Design review of the part built by this model. Coordinates are the model's own, in mm. Face numbers are marked on the shaded views. Give positions to 0.01 mm unless a question says otherwise; leave off trailing zeros. Write each loop counter-clockwise with the first axis right and the second up, starting at its lowest first coordinate (ties: lowest second). Pieces come first, ordered by that corner, then holes. Notation, with made-up numbers: M 40.25,43 L 49.25,43 A23 cw 49.25,60 Z; hole C -35.5,-14.5 d6. An arc over 180 degrees is marked long. Use one line per item in the form item = value. Start each with the question number.
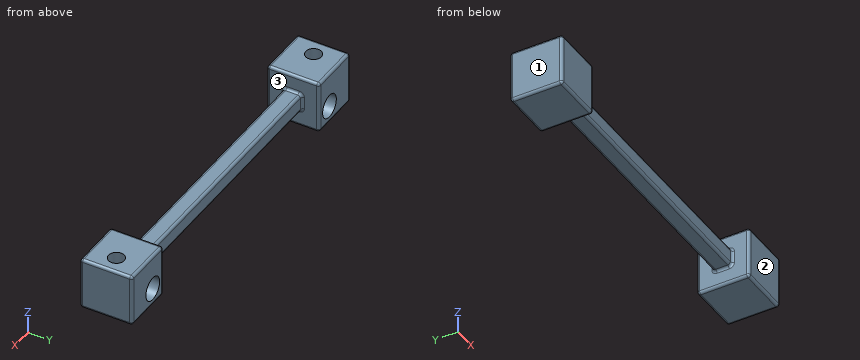
from build123d import *

# Parameters (mm, degrees)
BOSS_EXTRUDE1_START = -10
SKETCH1_W           = 30
SKETCH1_H           = 30
BOSS_EXTRUDE1_DEPTH = 30
SKETCH2_W           = 10
SKETCH2_H           = 10
BOSS_EXTRUDE2_DEPTH = 152.4
SKETCH3_W           = 6
SKETCH3_H           = 6
CUT_EXTRUDE1_DEPTH  = 152.4
SKETCH4_R           = 6.7
CUT_EXTRUDE2_DEPTH  = 15
SKETCH5_R           = 4.5
CUT_EXTRUDE3_DEPTH  = 15
FILLET3_R           = 1.5


with BuildPart() as part:
    # Sketch1 → Boss-Extrude1 (new body)
    with BuildSketch(Plane(origin=(0, 0, 0), x_dir=(0, 0, -1), z_dir=(1, 0, 0)).offset(BOSS_EXTRUDE1_START)):
        with Locations((15, 15)):
            Rectangle(SKETCH1_W, SKETCH1_H)
    boss_extrude1 = extrude(amount=BOSS_EXTRUDE1_DEPTH)

    # Sketch2 → Boss-Extrude2 (add)
    with BuildSketch(Plane(origin=(20, 0, 0), x_dir=(0, 0, -1), z_dir=(1, 0, 0))):
        with Locations((15, 15)):
            Rectangle(SKETCH2_W, SKETCH2_H)
    extrude(amount=BOSS_EXTRUDE2_DEPTH)

    # Sketch3 → Cut-Extrude1 (cut)
    with BuildSketch(Plane(origin=(172.4, 0, 0), x_dir=(0, 0, -1), z_dir=(1, 0, 0))):
        with Locations((15, 15)):
            Rectangle(SKETCH3_W, SKETCH3_H)
    extrude(amount=-CUT_EXTRUDE1_DEPTH, mode=Mode.SUBTRACT)

    # Sketch4 → Cut-Extrude2 (cut)
    with BuildSketch(Plane(origin=(0, 30, 0), x_dir=(1, 0, 0), z_dir=(0, 1, 0))):
        with Locations(Location((10, 20, 0), (0, 0, 270))):
            Circle(SKETCH4_R)
    cut_extrude2 = extrude(amount=-CUT_EXTRUDE2_DEPTH, mode=Mode.SUBTRACT)

    # Sketch5 → Cut-Extrude3 (cut)
    with BuildSketch(Plane.XY):
        with Locations((0, 15)):
            Circle(SKETCH5_R)
    cut_extrude3 = extrude(amount=-CUT_EXTRUDE3_DEPTH, mode=Mode.SUBTRACT)

    # Mirror1: Boss-Extrude1, Cut-Extrude2, Cut-Extrude3 across plane
    add(boss_extrude1.mirror(Plane(origin=(96.2, 0, 0), x_dir=(0, 0, 1), z_dir=(1, 0, 0))))
    add(cut_extrude2.mirror(Plane(origin=(96.2, 0, 0), x_dir=(0, 0, 1), z_dir=(1, 0, 0))), mode=Mode.SUBTRACT)
    add(cut_extrude3.mirror(Plane(origin=(96.2, 0, 0), x_dir=(0, 0, 1), z_dir=(1, 0, 0))), mode=Mode.SUBTRACT)

    # Fillet3
    fillet3_edges = [part.edges().sort_by_distance(p)[0] for p in [
        (20, 30, -15),
        (20, 15, 0),
        (20, 0, -15),
        (-10, 30, -15),
        (20, 15, -30),
        (-10, 15, 0),
        (20, 15, -10),
        (96.2, 20, -10),
        (20, 10, -15),
        (96.2, 10, -10),
        (20, 15, -20),
        (96.2, 10, -20),
        (20, 20, -15),
        (96.2, 20, -20),
        (172.4, 15, -10),
        (172.4, 10, -15),
        (172.4, 15, -20),
        (172.4, 20, -15),
        (-10, 0, -15),
        (187.4, 0, 0),
        (172.4, 0, -15),
        (187.4, 0, -30),
        (172.4, 15, -30),
        (187.4, 30, -30),
        (202.4, 30, -15),
        (187.4, 30, 0),
        (202.4, 15, 0),
        (202.4, 0, -15),
        (202.4, 15, -30),
        (172.4, 15, 0),
        (172.4, 30, -15),
        (5, 0, 0),
        (5, 30, 0),
        (5, 30, -30),
        (5, 0, -30),
        (-10, 15, -30),
    ]]
    fillet(fillet3_edges, radius=FILLET3_R)


solid = part.part
1. Clearance check with flat-ended pins moving along their axes: pin 1 Ø2 at (x, z) = (20, -7) entering from +Y; pin 2 Ø1.8 at (x, z) = (123.5, -16) entering from -Y; pin 3 Ø4.5 at (x, y) = (1.5, 15) entering from +Z. State where each tip first meets the part, or that it passes through.
2. We need section A-A (y = 24.5). State the section outline as (x, z) points.
3. To check wall thickness, follow L1, parallel to X at y = 24.25, z = -20; L2, parallel to Y at x = 92, z = -14.5; L3, parallel to X at y = 8.75, z = -23.5. State the ranges of each line that lie inside material, in increasing order.
4. Draft analysis for pull direction X (two halves, no side actions). For the marked faces 1, 2 and 3, state which applies: pulls with the +X half, pulls with the -X half, needs draft (parallel to the pull), parting line crosses it, or undercut.
5. We need section D-D (x = 10). State the section outline as (y, z) points, and give its area (3 significant figures).
6. We need section B-B (x = 86). State the section outline as (y, z) points, and give its area (3 significant figures).
7. We need section C-C (z = -24). State the section outline as (x, y) points, and give its area (3 significant figures).
Answer block:
q1.pin_1 = 29.91
q1.pin_2 = 10
q1.pin_3 = -15
q2.outline = M -10,-28.5 A1.5 ccw -8.5,-30 L 18.5,-30 A1.5 ccw 20,-28.5 L 20,-1.5 A1.5 ccw 18.5,0 L -8.5,0 A1.5 ccw -10,-1.5 Z; M 172.4,-28.5 A1.5 ccw 173.9,-30 L 200.9,-30 A1.5 ccw 202.4,-28.5 L 202.4,-1.5 A1.5 ccw 200.9,0 L 173.9,0 A1.5 ccw 172.4,-1.5 Z; hole C 10,-20 d13.4; hole C 182.4,-20 d13.4
q3.L1 = -10 to 3.3, 16.7 to 20, 172.4 to 175.7, 189.1 to 202.4
q3.L2 = 10 to 12, 18 to 20
q3.L3 = -10 to 20, 172.4 to 202.4
q4.face_1 = pulls with the -X half
q4.face_2 = needs draft
q4.face_3 = undercut
q5.outline = M 0,-28.5 A1.5 ccw 1.5,-30 L 28.5,-30 A1.5 ccw 30,-28.5 L 30,-26.7 L 15,-26.7 L 15,-13.3 L 30,-13.3 L 30,-1.5 A1.5 ccw 28.5,0 L 1.5,0 A1.5 ccw 0,-1.5 Z
q5.area = 697 mm^2
q6.outline = M 10,-18.5 A1.5 ccw 11.5,-20 L 18.5,-20 A1.5 ccw 20,-18.5 L 20,-11.5 A1.5 ccw 18.5,-10 L 11.5,-10 A1.5 ccw 10,-11.5 Z; hole M 12,-18 L 18,-18 L 18,-12 L 12,-12 Z
q6.area = 62.1 mm^2
q7.outline = M -10,1.5 A1.5 ccw -8.5,0 L 18.5,0 A1.5 ccw 20,1.5 L 20,28.5 A1.5 ccw 18.5,30 L 15.37,30 L 15.37,15 L 4.63,15 L 4.63,30 L -8.5,30 A1.5 ccw -10,28.5 Z; M 172.4,1.5 A1.5 ccw 173.9,0 L 200.9,0 A1.5 ccw 202.4,1.5 L 202.4,28.5 A1.5 ccw 200.9,30 L 187.77,30 L 187.77,15 L 177.03,15 L 177.03,30 L 173.9,30 A1.5 ccw 172.4,28.5 Z
q7.area = 1,470 mm^2
